Read the model definition and answer for the solid it produces. Units are mm, in the model's axes. A direction names the side the tool comes from. Coordinates: 2 decimals unless noted, no trailing zeros. Order: outer loops, then holes, each group sorted by start corner. A loop starts at its lowest first (then second) coordinate and runs counter-clockwise, first axis right, second up. Notation, with made-up numbers: M 3.5,-37.75 L 44.5,-37.75 A18 ccw 44.5,-2.75 Z; hole C -12.5,36.25 d3. An arc over 180 degrees is marked long. Put each result on its own line as item: value.
Autodesk Inventor part; units mm, degrees
ref_plane "YZ Plane" through (0, 0, 0) normal (1, 0, 0) x (0, 1, 0)
ref_plane "XZ Plane" through (0, 0, 0) normal (0, 1, 0) x (-1, 0, 0)
ref_plane "XY Plane" through (0, 0, 0) normal (0, 0, 1) x (1, 0, 0)
sketch "Sketch1" plane through (0, 0, 0) normal (0, 0, 1) x (1, 0, 0)
  line L0 (-39.5101, 21.6819) -> (-39.5101, 14.6819)
  line L1 (-39.5101, 14.6819) -> (-38.2601, 14.6819)
  line L2 (-38.2601, 14.6819) -> (-38.2601, 12.8819)
  line L3 (-38.2601, 12.8819) -> (-39.5101, 12.8819)
  line L4 (-39.5101, 12.8819) -> (-39.5101, 11.0819)
  line L5 (-39.5101, 11.0819) -> (-42.5101, 11.0819)
  line L6 (-42.5101, 11.0819) -> (-42.5101, 12.8819)
  line L7 (-42.5101, 12.8819) -> (-43.7601, 12.8819)
  line L8 (-43.7601, 12.8819) -> (-43.7601, 14.6819)
  line L9 (-43.7601, 14.6819) -> (-42.5101, 14.6819)
  line L10 (-42.5101, 14.6819) -> (-42.5101, 21.6819)
  line L11 (-42.5101, 21.6819) -> (-48.6101, 21.6819)
  line L12 (-48.6101, 21.6819) -> (-48.9101, 28.0819)
  line L13 (-48.9101, 28.0819) -> (-60.7101, 28.0819)
  line L14 (-60.7101, 28.0819) -> (-61.0101, 21.6819)
  line L15 (-61.0101, 21.6819) -> (-90.8101, 21.6819)
  line L16 (-90.8101, 21.6819) -> (-93.4912, 19.4321)
  line L17 (-93.4912, 19.4321) -> (-91.3057, 16.8276)
  line L18 (-91.3057, 16.8276) -> (-90.3482, 17.6311)
  line L19 (-90.3482, 17.6311) -> (-89.1912, 16.2522)
  line L20 (-89.1912, 16.2522) -> (-90.1487, 15.4487)
  line L21 (-90.1487, 15.4487) -> (-88.9917, 14.0698)
  line L22 (-88.9917, 14.0698) -> (-91.2898, 12.1415)
  line L23 (-91.2898, 12.1415) -> (-92.4469, 13.5203)
  line L24 (-92.4469, 13.5203) -> (-93.4044, 12.7169)
  line L25 (-93.4044, 12.7169) -> (-94.5614, 14.0957)
  line L26 (-94.5614, 14.0957) -> (-93.6039, 14.8992)
  line L27 (-93.6039, 14.8992) -> (-95.7894, 17.5038)
  line L28 (-95.7894, 17.5038) -> (-131.7932, -12.7071)
  line L29 (-131.7932, -12.7071) -> (-129.6078, -15.3116)
  line L30 (-129.6078, -15.3116) -> (-128.6502, -14.5082)
  line L31 (-128.6502, -14.5082) -> (-127.4932, -15.887)
  line L32 (-127.4932, -15.887) -> (-128.4508, -16.6905)
  line L33 (-128.4508, -16.6905) -> (-127.2937, -18.0694)
  line L34 (-127.2937, -18.0694) -> (-129.5919, -19.9978)
  line L35 (-129.5919, -19.9978) -> (-130.7489, -18.6189)
  line L36 (-130.7489, -18.6189) -> (-131.7064, -19.4224)
  line L37 (-131.7064, -19.4224) -> (-132.8635, -18.0435)
  line L38 (-132.8635, -18.0435) -> (-131.9059, -17.24)
  line L39 (-131.9059, -17.24) -> (-133.9788, -14.7696)
  line L40 (-133.9788, -14.7696) -> (-136.66, -17.0193)
  line L41 (-136.66, -17.0193) -> (-136.5205, -21.4818)
  arc A0 (-136.5205, -21.4818) -> (-134.5215, -23.4193) centre (-134.5215, -21.4193) ccw
  line L42 (-134.5215, -23.4193) -> (-120.7985, -23.4193)
  arc A1 (-120.7985, -23.4193) -> (-118.7994, -21.4818) centre (-120.7985, -21.4193) ccw
  line L43 (-118.7994, -21.4818) -> (-118.66, -17.0193)
  line L44 (-118.66, -17.0193) -> (-56.7602, -17.0193)
  line L45 (-56.7602, -17.0193) -> (-56.7602, -10.0193)
  line L46 (-56.7602, -10.0193) -> (-58.0102, -10.0193)
  line L47 (-58.0102, -10.0193) -> (-58.0102, -8.2193)
  line L48 (-58.0102, -8.2193) -> (-56.7602, -8.2193)
  line L49 (-56.7602, -8.2193) -> (-56.7602, -6.4193)
  line L50 (-56.7602, -6.4193) -> (-53.7602, -6.4193)
  line L51 (-53.7602, -6.4193) -> (-53.7602, -8.2193)
  line L52 (-53.7602, -8.2193) -> (-52.5102, -8.2193)
  line L53 (-52.5102, -8.2193) -> (-52.5102, -10.0193)
  line L54 (-52.5102, -10.0193) -> (-53.7602, -10.0193)
  line L55 (-53.7602, -10.0193) -> (-53.7602, -17.0193)
  line L56 (-53.7602, -17.0193) -> (2.24, -17.0193)
  line L57 (2.24, -17.0193) -> (2.24, -13.3193)
  line L58 (2.24, -13.3193) -> (9.24, -13.3193)
  line L59 (9.24, -13.3193) -> (9.24, -17.0193)
  line L60 (9.24, -17.0193) -> (22.885, -17.0193)
  line L61 (22.885, -17.0193) -> (23.185, -23.4193)
  line L62 (23.185, -23.4193) -> (34.985, -23.4193)
  line L63 (34.985, -23.4193) -> (35.285, -17.0193)
  line L64 (35.285, -17.0193) -> (41.385, -17.0193)
  line L65 (41.385, -17.0193) -> (41.385, -10.0193)
  line L66 (41.385, -10.0193) -> (40.135, -10.0193)
  line L67 (40.135, -10.0193) -> (40.135, -8.2193)
  line L68 (40.135, -8.2193) -> (41.385, -8.2193)
  line L69 (41.385, -8.2193) -> (41.385, -6.4193)
  line L70 (41.385, -6.4193) -> (44.385, -6.4193)
  line L71 (44.385, -6.4193) -> (44.385, -8.2193)
  line L72 (44.385, -8.2193) -> (45.635, -8.2193)
  line L73 (45.635, -8.2193) -> (45.635, -10.0193)
  line L74 (45.635, -10.0193) -> (44.385, -10.0193)
  line L75 (44.385, -10.0193) -> (44.385, -17.0193)
  line L76 (44.385, -17.0193) -> (50.485, -17.0193)
  line L77 (50.485, -17.0193) -> (50.785, -23.4193)
  line L78 (50.785, -23.4193) -> (62.585, -23.4193)
  line L79 (62.585, -23.4193) -> (62.885, -17.0193)
  line L80 (62.885, -17.0193) -> (64.695, -17.0193)
  line L81 (64.695, -17.0193) -> (64.695, -3.7245)
  line L82 (64.695, -3.7245) -> (64.695, -0.6157)
  line L83 (64.695, -0.6157) -> (64.695, 16.6819)
  arc A2 (64.695, 16.6819) -> (59.695, 21.6819) centre (59.695, 16.6819) ccw
  line L84 (59.695, 21.6819) -> (-21.0101, 21.6819)
  line L85 (-21.0101, 21.6819) -> (-21.3101, 28.0819)
  line L86 (-21.3101, 28.0819) -> (-33.1101, 28.0819)
  line L87 (-33.1101, 28.0819) -> (-33.4101, 21.6819)
  line L88 (-33.4101, 21.6819) -> (-39.5101, 21.6819)
  point P0 (0, 0)
  point P1 (0, 0)
extrude "Extrusion1" add sketch "Sketch1" along normal blind 6
properties part number "boardCaseSide"
Q1. A tool of negligible diameter and unlimited length cuts with its end or side. For faces 4 (the face through (35.133, -20.264, 2.958)), 5 (the face through (-33.258, 24.927, 2.958)), 6 (the face through (57, -23.419, 3)), from which of +Z, -Z, +X, -X, +Y, -Y can it reach the whole face along a straight path? Write none if from no direction.
Answers below:
face 4: +Z, -Z, -Y
face 5: +Z, -Z, +Y
face 6: +Z, -Z, +X, -X, -Y
Q2. For a pull along X with two mould halves and no side action, classify faces 1 (the face through (20, 21.682, 3)), 2 (the face through (16, -17.019, 3)), 3 (the face through (64.695, 0, 3)) as +X half, -X half, draft (parallel to the pull), parting line (faces both ways), or undercut.
Answers below:
face 1: draft
face 2: undercut
face 3: +X half
Q3. Given pin 1 (1.8 mm diameter, centred on y = 17.5, z = 2.5, fed in from -X); pin 2 (1.5 mm diameter, centred on x = -55, z = 4.5, fed in from -Y); pin 3 (1 mm diameter, centred on x = 45, z = 3, fed in from +Y), each flat-ended and moving along its own axis, determine where each tip first touches the part or whether it passes through.
Answers below:
pin 1: stops at x = -96.87
pin 2: stops at y = -6.42
pin 3: stops at y = 21.68
Q4. Find section B-B on y = 1. Write down the section's boundary in (x, z) (3 decimals).
Answers below:
outline: M -115.458,0 L 64.695,0 L 64.695,6 L -115.458,6 Z
Q5. Find section A-A on x = 37.5. Write down the section's boundary in (y, z).
Answers below:
outline: M -17.02,0 L 21.68,0 L 21.68,6 L -17.02,6 Z
Q6. Consider line 1 along X through (y, z) = (-7, 2.4) (3 decimals); line 2 along X through (y, z) = (-13.5, 3.2) (3 decimals); line 3 along Y through (x, z) = (-128, 1.4). Determine where each line is inside the solid, lowest interval first.
Answers below:
line 1: x = -124.992 to -56.76, -53.76 to 41.385, 44.385 to 64.695
line 2: x = -131.128 to -56.76, -53.76 to 2.24, 9.24 to 41.385, 44.385 to 64.695
line 3: y = -23.42 to -18.66, -17.23 to -16.31, -15.28 to -9.52
